Could you check a few things on this drawing? It's one solid part, dimensions in mm from its lowest x, y, z. A direction names the side the tool comes from. Coordinates: 2 decimals unless noted, no trailing zeros. Order: outer loops, then holes, each group sorted by start corner. A loop starts at its lowest first (then second) coordinate and runs counter-clockwise, first axis right, second up. Notation, with made-up numbers: (-25.5, 79.25) - (12.5, 79.25) arc R17 ccw to (12.5, 111.25) - close; hole circle Ø10 at (50.25, 50). An arc over 180 degrees is marked (long way). Return JSON: item names as keys, results as strings. Group by question number.
1) If we mould it in two halves opening along X, with no side actions, what happens to the marked faces 5, 6 and 7? For each: pulls with the +X half, pulls with the -X half, needs draft (parallel to the pull), parting line crosses it, or undercut.
2) Imagine slicing it at B-B (z = 8.5). Write out the boundary of the cut face in (x, y).
3) Imagine slicing it at D-D (x = 6.05). Write out the boundary of the cut face in (y, z), and give its area (3 significant figures).
4) Imagine slicing it at C-C (z = 7). Write out the boundary of the cut face in (x, y).
5) If I drill on line 1 along X through (y, z) = (1.65, 8.5); line 2 along Z through (x, y) = (15.75, 4.25); line 3 along X through (y, z) = (7.25, 12.75), over which ranges is the centre line in solid material (lowest first)?
6) Imagine slicing it at A-A (x = 27.96). Write out the boundary of the cut face in (y, z), and give its area (3 significant figures).
7) For pin 1 Ø6.5 at (x, z) = (16.5, 6.5) entering from -Y; pin 2 Ø0.6 at (y, z) = (1.5, 13) entering from +X; pin 3 Ø2.5 at (x, z) = (1.84, 8.5) entering from +Y, each with a flat end and sliding along its axis, tell me the tip position at first contact or that it passes through.
8) Which directions (+Z, -Z, +X, -X, +Y, -Y) give clear straight access to the entire face, cutting with the end or side of a thin tool? Please do the marked faces 1, 2, 3 and 4.
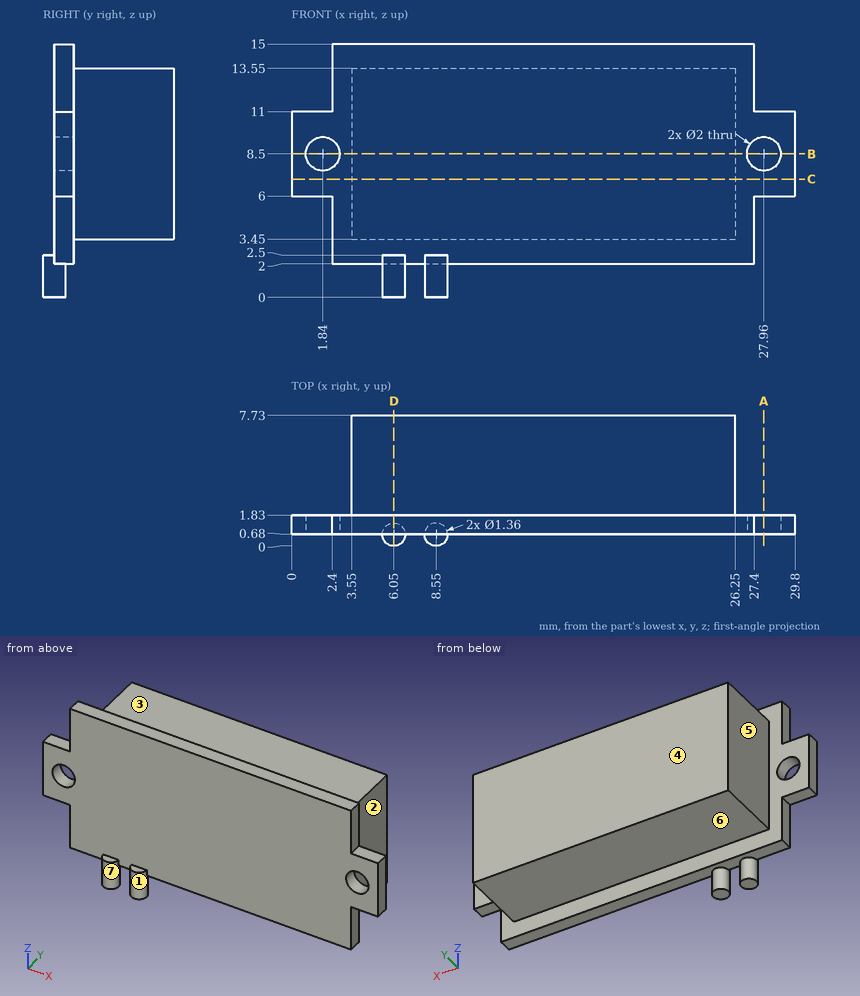
Calculated:
{
 "1": {"face 5": "pulls with the -X half", "face 6": "needs draft", "face 7": "undercut"},
 "2": {"outline": "(0, 0.68) - (0.84, 0.68) - (0.84, 1.83) - (0, 1.83) - close; (2.84, 0.68) - (26.96, 0.68) - (26.96, 1.83) - (26.25, 1.83) - (26.25, 7.73) - (3.55, 7.73) - (3.55, 1.83) - (2.84, 1.83) - close; (28.96, 0.68) - (29.8, 0.68) - (29.8, 1.83) - (28.96, 1.83) - close"},
 "3": {"outline": "(0, 0) - (1.36, 0) - (1.36, 2) - (1.83, 2) - (1.83, 3.45) - (7.73, 3.45) - (7.73, 13.55) - (1.83, 13.55) - (1.83, 15) - (0.68, 15) - (0.68, 2.5) - (0, 2.5) - close", "area": "77.6 mm2"},
 "4": {"outline": "(0, 0.68) - (29.8, 0.68) - (29.8, 1.83) - (26.25, 1.83) - (26.25, 7.73) - (3.55, 7.73) - (3.55, 1.83) - (0, 1.83) - close"},
 "5": {"line 1": "0 to 0.84, 2.84 to 26.96, 28.96 to 29.8", "line 2": "3.45 to 13.55", "line 3": "3.55 to 26.25"},
 "6": {"outline": "(0.68, 6) - (1.83, 6) - (1.83, 7.5) - (0.68, 7.5) - close; (0.68, 9.5) - (1.83, 9.5) - (1.83, 11) - (0.68, 11) - close", "area": "3.45 mm2"},
 "7": {"pin 1": "y = 0.68", "pin 2": "x = 27.4", "pin 3": "y = 1.83"},
 "8": {"face 1": "-Z", "face 2": "+Z, -Z, +X, +Y", "face 3": "+Z, +X, -X, +Y", "face 4": "+Z, -Z, +X, -X, +Y"}
}
